```python
from build123d import *

# Parameters (mm, degrees)
F0_W     = 8
F0_H     = 7.2
F1_DEPTH = 5.4
F2_R     = 2.4
F3_DEPTH = 6
F4_R     = 1.25
F5_DEPTH = 10
F6_W     = 0.5
F6_H     = 1.4
F7_DEPTH = 3
F8_W     = 0.5
F8_H     = 1.4
F9_DEPTH = 4.5


with BuildPart() as f1:
    # F0 (on Front) → F1 (new body)
    with BuildSketch(Plane.XZ):
        with Locations((4, 3.6)):
            Rectangle(F0_W, F0_H)
    extrude(amount=F1_DEPTH)

    # F2 (on face) → F3 (join)
    with BuildSketch(Plane.XY.offset(7.2)):
        with Locations((4, -2.7)):
            Circle(F2_R)
    extrude(amount=F3_DEPTH)

    # F4 (on face) → F5 (join)
    with BuildSketch(Plane.XY.offset(13.2)):
        with Locations((4, -2.7)):
            Circle(F4_R)
    extrude(amount=F5_DEPTH)

    # F6 (on face) → F7 (join)
    with BuildSketch(Plane(origin=(0, 0, 0), x_dir=(1, 0, 0), z_dir=(0, 0, -1))):
        with Locations((1.55, 2.7)):
            Rectangle(F6_W, F6_H)
        with Locations((6.45, 2.7)):
            Rectangle(F6_W, F6_H)
    extrude(amount=F7_DEPTH)

    # F8 (on face) → F9 (join)
    with BuildSketch(Plane(origin=(0, 0, 0), x_dir=(1, 0, 0), z_dir=(0, 0, -1))):
        with Locations((4, 2.7)):
            Rectangle(F8_W, F8_H)
    extrude(amount=F9_DEPTH)


solid = f1.part
```
Work out the finished part from the listing and answer in its coordinate system (mm). A direction names the side the tool comes from. Round coordinates to 2 decimals unless told otherwise and drop trailing zeros. Write each loop counter-clockwise with the first axis right and the second up, starting at its lowest first coordinate (ties: lowest second). Pieces come first, ordered by that corner, then holes.
1) A cutting plane is placed at B-B on x = 4. Determine the outline of the cut face in (y, z).
2) A cutting plane is placed at D-D on x = 7.25. Determine the outline of the cut face in (y, z), and give its area (3 significant figures).
3) Consider probe 1 along Z at (x, y) = (6, -3.35); probe 2 along Z at (x, y) = (1, -2.25); probe 3 along Y at (x, z) = (6.25, -2.75). Determine where each line is inside the solid, lowest interval first.
4) Flat-ended cylindrical pins translate along their axes: P1, Ø0.7, axis at y = -2.5, z = -2.5, coming from the -X side; P2, Ø0.6, axis at x = 1.5, y = -2.5, coming from the -Z side; P3, Ø1, axis at x = 5, y = -1, coming from the -Z side. Find the tip coordinate at first contact, or state that the pin passes through.
5) A cutting plane is placed at C-C on z = 20.5. Determine the outline of the cut face in (x, y), and give its area (3 significant figures).
6) Determine the mould class of faces 6 (the face through (1.8, -3, -1)), 7 (the face through (0, -3, 4)), 8 (the face through (3.48, -5.043, 10.158)) for opening direction X: pulls with the +X half, pulls with the -X half, needs draft (parallel to the pull), parting line crosses it, or undercut.
7) Which of the six approach directions +Z, -Z, +X, -X, +Y, -Y give full straight-line access (tool end or side, diameter ignored) to faces 1 (the face through (6.7, -3, -1)), 2 (the face through (1.3, -3, -1)), 3 (the face through (5.155, -3.179, 18.13)), 4 (the face through (4.25, -3, -2)), 5 (the face through (8, -3, 4))?
8) A cutting plane is placed at A-A on y = -2.7. Determine the outline of the cut face in (x, z), and give its area (3 significant figures).
Entries:
1. outline: (-5.4, 0) - (-3.4, 0) - (-3.4, -4.5) - (-2, -4.5) - (-2, 0) - (0, 0) - (0, 7.2) - (-0.3, 7.2) - (-0.3, 13.2) - (-1.45, 13.2) - (-1.45, 23.2) - (-3.95, 23.2) - (-3.95, 13.2) - (-5.1, 13.2) - (-5.1, 7.2) - (-5.4, 7.2) - close
2. outline: (-5.4, 0) - (0, 0) - (0, 7.2) - (-5.4, 7.2) - close
2. area: 38.9 mm2
3. probe 1: z = 0 to 13.2
3. probe 2: z = 0 to 7.2
3. probe 3: y = -3.4 to -2
4. P1: stops at x = 1.3
4. P2: stops at z = -3
4. P3: stops at z = 0
5. outline: circle Ø2.5 at (4, -2.7)
5. area: 4.91 mm2
6. face 6: undercut
6. face 7: pulls with the -X half
6. face 8: parting line crosses it
7. face 1: -Z, +X, +Y, -Y
7. face 2: -Z, -X, +Y, -Y
7. face 3: +Z
7. face 4: -Z, +Y, -Y
7. face 5: +Z, -Z, +X, +Y, -Y
8. outline: (0, 0) - (1.3, 0) - (1.3, -3) - (1.8, -3) - (1.8, 0) - (3.75, 0) - (3.75, -4.5) - (4.25, -4.5) - (4.25, 0) - (6.2, 0) - (6.2, -3) - (6.7, -3) - (6.7, 0) - (8, 0) - (8, 7.2) - (6.4, 7.2) - (6.4, 13.2) - (5.25, 13.2) - (5.25, 23.2) - (2.75, 23.2) - (2.75, 13.2) - (1.6, 13.2) - (1.6, 7.2) - (0, 7.2) - close
8. area: 117 mm2
